Design review of the part built by this model. Coordinates are the model's own, in mm. Face numbers are marked on the shaded views. Coordinates: 2 decimals unless noted, no trailing zeros. Loops run counter-clockwise (first coordinate to the right, second up) from the corner with the lowest first, then second, coordinate; pieces in that order, holes last. Notation, with made-up numbers: (80, -3.5) - (105, -3.5) arc R14 ccw to (105, 20.5) - close; hole circle Ø3 at (59.25, 23). An arc over 180 degrees is marked (long way). Answer in a Markdown table with one row per item. Add a question column.
(1) The part is to be moulded in two halves that separate along Y. For the marked faces 1, 2 and 3, say which applies: released by +Y, released by -Y, zero draft, split by the parting line, or undercut.
(2) We need section A-A, the plane z = 3.75. Write out the cut boundary in (x, y).
(3) We need section B-B, the plane y = 15. Write out the cut boundary in (x, z), plus the area to 3 significant figures.
(4) Clearance check with flat-ended pins moving along their axes: pin 1 (17 mm diameter, centred on x = 9, y = 24, fed in from -Z); pin 2 (1 mm diameter, centred on x = 14.5, z = 1.5, fed in from -Y); pin 3 (2.5 mm diameter, centred on y = 1, z = -1, fed in from +X). State where each tip first meets the part, or that it passes through.
(5) To check wall thickness, follow L1, parallel to Z at x = -6.35, y = 1.15; L2, parallel to Z at x = 24, y = 32; L3, parallel to Y at x = -4, z = 7.25. State the ranges of each line that lie inside material, in increasing order. Write a range as [from, to].
(6) We need section C-C, the plane x = 24. Write out the cut boundary in (y, z), plus the area to 3 significant figures.
(7) We need section D-D, the plane x = 0. Write out the cut boundary in (y, z).
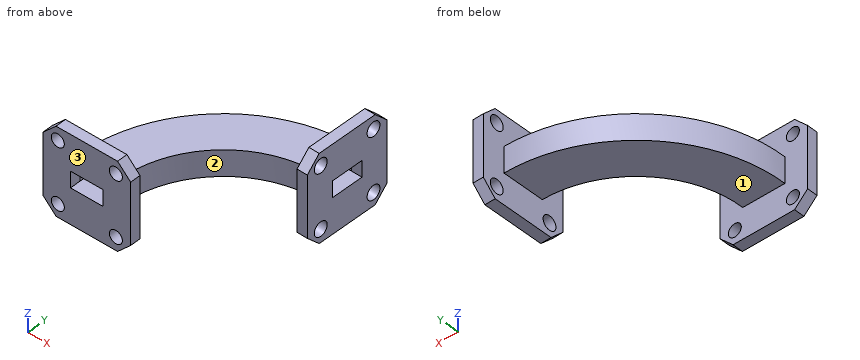
from build123d import *

# Parameters (mm, degrees)
SKETCH1_W           = 19.177
SKETCH1_H           = 19.177
BOSS_EXTRUDE1_DEPTH = 2.286
SKETCH2_R           = 1.4224
SKETCH2_W           = 7.112
SKETCH2_H           = 3.556
CUT_EXTRUDE1_DEPTH  = 2.286
SKETCH3_W           = 9.2202
SKETCH3_H           = 5.6642
SKETCH3_W_2         = 7.112
SKETCH3_H_2         = 3.556
SKETCH5_W           = 19.177
SKETCH5_H           = 19.177
SKETCH5_R           = 1.5494
SKETCH5_W_2         = 3.556
SKETCH5_H_2         = 7.112
BOSS_EXTRUDE2_DEPTH = 2.286
CHAMFER1_SIZE       = 2.8575


with BuildPart() as part:
    # Sketch1 → Boss-Extrude1 (new body)
    with BuildSketch(Plane(origin=(0, 0, 0), x_dir=(1, 0, 0), z_dir=(0, 1, 0))):
        Rectangle(SKETCH1_W, SKETCH1_H)
    extrude(amount=BOSS_EXTRUDE1_DEPTH)

    # Sketch2 → Cut-Extrude1 (cut)
    with BuildSketch(Plane(origin=(0, 2.286, 0), x_dir=(1, 0, 0), z_dir=(0, 1, 0))):
        with Locations((-6.35, 6.731)):
            Circle(SKETCH2_R)
        with Locations((6.35, 6.731)):
            Circle(SKETCH2_R)
        with Locations((6.35, -6.731)):
            Circle(SKETCH2_R)
        with Locations((-6.35, -6.731)):
            Circle(SKETCH2_R)
        Rectangle(SKETCH2_W, SKETCH2_H)
    extrude(amount=-CUT_EXTRUDE1_DEPTH, mode=Mode.SUBTRACT)

    # Sweep1: sweep along a path in Sketch4
    with BuildLine(Plane.XY) as sweep1_path:
        ThreePointArc((4.6101, 2.286), (11.285803016, 18.770237549), (27.7241, 25.558277811))
    # Sketch3 → Sweep1 (sweep)
    with BuildSketch(Plane(origin=(0, 2.286, 0), x_dir=(1, 0, 0), z_dir=(0, 1, 0))):
        Rectangle(SKETCH3_W, SKETCH3_H)
        Rectangle(SKETCH3_W_2, SKETCH3_H_2, mode=Mode.SUBTRACT)
    sweep(path=sweep1_path.line)

    # Sketch5 → Boss-Extrude2 (add)
    with BuildSketch(Plane(origin=(27.255255403, -0.490558544, 0), x_dir=(0, 0, -1), z_dir=(0.999838063, -0.017995763, 0))):
        with Locations((0, 30.663155305)):
            Rectangle(SKETCH5_W, SKETCH5_H)
        with Locations((-6.731, 37.013155305)):
            Circle(SKETCH5_R, mode=Mode.SUBTRACT)
        with Locations((6.731, 37.013155305)):
            Circle(SKETCH5_R, mode=Mode.SUBTRACT)
        with Locations((-6.731, 24.313155305)):
            Circle(SKETCH5_R, mode=Mode.SUBTRACT)
        with Locations((6.731, 24.313155305)):
            Circle(SKETCH5_R, mode=Mode.SUBTRACT)
        with Locations((0, 30.663155305)):
            Rectangle(SKETCH5_W_2, SKETCH5_H_2, mode=Mode.SUBTRACT)
    extrude(amount=BOSS_EXTRUDE2_DEPTH)

    # Chamfer1
    chamfer1_edges = [part.edges().sort_by_distance(p)[0] for p in [
        (29.122429541, 39.734009377, 9.5885),
        (28.777324802, 20.56011484, 9.5885),
        (28.777324802, 20.56011484, -9.5885),
        (29.122429541, 39.734009377, -9.5885),
        (-9.5885, 1.143, -9.5885),
        (9.5885, 1.143, -9.5885),
        (9.5885, 1.143, 9.5885),
        (-9.5885, 1.143, 9.5885),
    ]]
    chamfer(chamfer1_edges, length=CHAMFER1_SIZE)


solid = part.part
Responses:
| question | item | result |
|---|---|---|
| 1 | face 1 | zero draft |
| 1 | face 2 | undercut |
| 1 | face 3 | released by -Y |
| 2 | outline | (-9.59, 0) - (9.59, 0) - (9.59, 2.29) - (-9.59, 2.29) - close; (27.63, 20.58) - (29.92, 20.54) - (30.27, 39.71) - (27.98, 39.75) - close |
| 3 | outline | (-2.12, -2.83) - (8.26, -2.83) - (8.26, 2.83) - (-2.12, 2.83) - close; hole (-0.97, -1.78) - (7.02, -1.78) - (7.02, 1.78) - (-0.97, 1.78) - close |
| 3 | area | 30.4 mm2 |
| 4 | pin 1 | stops at z = -2.83 |
| 4 | pin 2 | stops at y = 21.11 |
| 4 | pin 3 | stops at x = 9.59 |
| 5 | L1 | z = [-9.59, -8.15], [-5.31, 5.31], [8.15, 9.59] |
| 5 | L2 | z = [-2.83, -1.78], [1.78, 2.83] |
| 5 | L3 | y = [0, 2.29] |
| 6 | outline | (25.28, -2.83) - (34.58, -2.83) - (34.58, 2.83) - (25.28, 2.83) - close; hole (26.34, -1.78) - (33.52, -1.78) - (33.52, 1.78) - (26.34, 1.78) - close |
| 6 | area | 27.2 mm2 |
| 7 | outline | (0, -9.59) - (2.29, -9.59) - (2.29, -2.83) - (19.18, -2.83) - (19.18, 2.83) - (2.29, 2.83) - (2.29, 9.59) - (0, 9.59) - (0, 1.78) - (17.03, 1.78) - (17.03, -1.78) - (0, -1.78) - close |
